Work out the finished part from the listing and answer in its coordinate system (mm). A direction names the side the tool comes from. Round coordinates to 2 decimals unless told otherwise and drop trailing zeros. Order: outer loops, then holes, each group sorted by start corner. A loop starts at its lowest first (then second) coordinate and runs counter-clockwise, first axis right, second up. Notation, with made-up numbers: (69, 78.25) - (126, 78.25) arc R15 cw to (126, 102.25) - close; hole circle Ø3 at (75, 77). An arc over 180 degrees is marked (long way). Use one line per item in the form item = value. Start each with the question number.
Q1. Given P1, Ø5, axis at x = 2, z = 2.5, coming from the -Y side; P2, Ø5, axis at x = 5, y = 11.5, coming from the -Z side; P3, Ø5, axis at x = 5, y = -15, coming from the +Z side, each flat-ended and moving along its own axis, determine where each tip first touches the part or whether it passes through.
Q2. Which of the six approach directions +Z, -Z, +X, -X, +Y, -Y give full straight-line access (tool end or side, diameter ignored) to faces 4 (the cylindrical face through (2.46, 2.32, 10.06)), 5 (the flat face through (7.3, 10, 9.92)), 6 (the flat face through (5, -11, 3)), 7 (the flat face through (5, -37.66, 12)), 8 (the flat face through (7.3, -32.5, 9.92))?
Q3. Find the intervals of material crossed by line 1 (Y direction, x = 7.5, z = 11.5); line 2 (Y direction, x = 6.5, z = 5); line 3 (Y direction, x = 6.5, z = 12.5), in increasing order. Write a range as [from, to].
Q4. The part is cut by section D-D on x = 9. Determine the outline of the cut face in (y, z).
Q5. The part is cut by section C-C on y = -33.5. Determine the outline of the cut face in (x, z), plus the area to 3 significant figures.
Q6. The part is cut by section B-B on x = 2. Determine the outline of the cut face in (y, z), plus the area to 3 significant figures.
Q7. The part is cut by section A-A on z = 3.75. Determine the outline of the cut face in (x, y), plus the area to 4 significant figures.
Q8. For a pull along X with two mould halves and no side action, classify faces 1 (the flat face through (10, -11.6, 2.6)), 2 (the cylindrical face through (4.75, -34.47, 12.5)), 3 (the flat face through (0, -11.6, 2.6)) as +X half, -X half, draft (parallel to the pull), parting line (faces both ways), or undercut.
from build123d import *

# Parameters (mm, degrees)
SKETCH1_W                  = 26.40999036
SKETCH1_H                  = 14.9999954
BOSS_EXTRUDE1_DEPTH        = 10.0000054
SKETCH2_W                  = 12.0000014
SKETCH2_H                  = 11.25000036
CUT_EXTRUDE1_DEPTH         = 11.0000054
SKETCH3_W                  = 9.9199954
SKETCH3_H                  = 10.16
CUT_EXTRUDE2_DEPTH         = 11.0000054
M3_5_CLEARANCE_HOLE1_D     = 3.81
M3_5_CLEARANCE_HOLE1_DEPTH = 5.08


with BuildPart() as part:
    # Sketch1 → Boss-Extrude1 (new body)
    with BuildSketch(Plane(origin=(0, 0, 0), x_dir=(0, -1, 0), z_dir=(-1, 0, 0))):
        with Locations((-1.95499482, 7.4999977)):
            Rectangle(SKETCH1_W, SKETCH1_H)
    boss_extrude1 = extrude(amount=-BOSS_EXTRUDE1_DEPTH)

    # Sketch2 → Cut-Extrude1 (cut, through all)
    with BuildSketch(Plane(origin=(10.0000054, 0, 0), x_dir=(0, 0, -1), z_dir=(1, 0, 0))):
        with Locations((-8.9999947, -5.62500018)):
            Rectangle(SKETCH2_W, SKETCH2_H)
    cut_extrude1 = extrude(amount=-CUT_EXTRUDE1_DEPTH, mode=Mode.SUBTRACT)

    # Sketch3 → Cut-Extrude2 (cut, through all)
    with BuildSketch(Plane(origin=(10.0000054, 0, 0), x_dir=(0, 0, -1), z_dir=(1, 0, 0))):
        with Locations((-4.9599977, 10.07999)):
            Rectangle(SKETCH3_W, SKETCH3_H)
    cut_extrude2 = extrude(amount=-CUT_EXTRUDE2_DEPTH, mode=Mode.SUBTRACT)

    # M3.5 Clearance Hole1
    with Locations(Plane(origin=(0, 0, 9.9199954), x_dir=(-1, 0, 0), z_dir=(0, 0, -1))):
        with Locations((-4.99999, 10.07999)):
            m3_5_clearance_hole1 = Hole(M3_5_CLEARANCE_HOLE1_D / 2, depth=M3_5_CLEARANCE_HOLE1_DEPTH)

    # Sketch6 → Ø1.2 (1.2) Diameter Hole1 (revolve, cut)
    with BuildSketch(Plane(origin=(0, 2.50000008, 9.4881954), x_dir=(0, 0, 1), z_dir=(0, 1, 0))):
        Polygon((0, 0), (0, 5.360506413), (0.60000007, 4.99999), (0.60000007, 0), align=None)
    f_1_2_1_2_diameter_hole1 = revolve(axis=Axis((-6.35, 2.50000008, 9.4881954), (1, 0, 0)), mode=Mode.SUBTRACT)

    # Mirror1: Boss-Extrude1, Cut-Extrude1, Cut-Extrude2, M3.5 Clearance Hole1, Ø1.2 (1.2) Diameter Hole1 across plane
    add(boss_extrude1.mirror(Plane(origin=(0, -11.25000036, 0), x_dir=(0, 0, 1), z_dir=(0, -1, 0))))
    add(cut_extrude1.mirror(Plane(origin=(0, -11.25000036, 0), x_dir=(0, 0, 1), z_dir=(0, -1, 0))), mode=Mode.SUBTRACT)
    add(cut_extrude2.mirror(Plane(origin=(0, -11.25000036, 0), x_dir=(0, 0, 1), z_dir=(0, -1, 0))), mode=Mode.SUBTRACT)
    add(m3_5_clearance_hole1.mirror(Plane(origin=(0, -11.25000036, 0), x_dir=(0, 0, 1), z_dir=(0, -1, 0))), mode=Mode.SUBTRACT)
    add(f_1_2_1_2_diameter_hole1.mirror(Plane(origin=(0, -11.25000036, 0), x_dir=(0, 0, 1), z_dir=(0, -1, 0))), mode=Mode.SUBTRACT)


solid = part.part
Found:
q1.P1 = -27.5
q1.P2 = 9.92
q1.P3 = 3
q2.face_4 = -X
q2.face_5 = -Z, +X, -X, +Y
q2.face_6 = +Z, +X, -X
q2.face_7 = +Z, -Z, +X, -X, -Y
q2.face_8 = -Z, +X, -X, -Y
q3.line_1 = [-37.66, -22.5], [0, 15.16]
q3.line_2 = [-27.5, -22.5], [0, 5]
q3.line_3 = [-37.66, -33.75], [-31.41, -22.5], [0, 8.91], [11.25, 15.16]
q4.outline = (-37.66, 9.92) - (-27.5, 9.92) - (-27.5, 0) - (5, 0) - (5, 9.92) - (15.16, 9.92) - (15.16, 15) - (0, 15) - (0, 3) - (-22.5, 3) - (-22.5, 15) - (-37.66, 15) - close
q5.outline = (0, 9.92) - (3.33, 9.92) - (3.33, 15) - (0, 15) - close; (6.67, 9.92) - (10, 9.92) - (10, 15) - (6.67, 15) - close
q5.area = 33.9 mm²
q6.outline = (-37.66, 9.92) - (-27.5, 9.92) - (-27.5, 0) - (5, 0) - (5, 9.92) - (15.16, 9.92) - (15.16, 15) - (0, 15) - (0, 3) - (-22.5, 3) - (-22.5, 15) - (-37.66, 15) - close; hole circle Ø1.2 at (-25, 9.49); hole circle Ø1.2 at (2.5, 9.49)
q6.area = 318 mm²
q7.outline = (0, -27.5) - (10, -27.5) - (10, -22.5) - (0, -22.5) - close; (0, 0) - (10, 0) - (10, 5) - (0, 5) - close
q7.area = 100.0 mm²
q8.face_1 = +X half
q8.face_2 = undercut
q8.face_3 = -X half
